```python
from build123d import *

# Parameters (mm, degrees)
F1_DEPTH = 5.842


with BuildPart() as f1:
    # F0 (on Top) → F1 (new body)
    with BuildSketch(Plane.XY):
        with BuildLine():
            Line((95.142507, 46.804437), (-38.207493, 46.804437))
            ThreePointArc((-38.207493, 46.804437), (-42.697621, 44.944565), (-44.557493, 40.454437))
            Line((-44.557493, 40.454437), (-44.557493, 27.754437))
            ThreePointArc((-44.557493, 27.754437), (-42.697621, 23.264309), (-38.207493, 21.404437))
            Line((-38.207493, 21.404437), (95.142507, 21.404437))
            Line((95.142507, 21.404437), (95.142507, 8.704437))
            Line((95.142507, 8.704437), (-38.207493, 8.704437))
            ThreePointArc((-38.207493, 8.704437), (-42.697621, 6.844565), (-44.557493, 2.354437))
            Line((-44.557493, 2.354437), (-44.557493, -10.345563))
            ThreePointArc((-44.557493, -10.345563), (-42.697621, -14.835691), (-38.207493, -16.695563))
            Line((-38.207493, -16.695563), (95.142507, -16.695563))
            Line((95.142507, -16.695563), (95.142507, -29.395563))
            Line((95.142507, -29.395563), (101.492507, -29.395563))
            Line((101.492507, -29.395563), (101.492507, 59.504437))
            Line((101.492507, 59.504437), (95.142507, 59.504437))
            Line((95.142507, 59.504437), (95.142507, 46.804437))
        make_face()
    extrude(amount=F1_DEPTH)


solid = f1.part
```
Geometry check sheet. Reference: the model listing, model coordinates, mm. A direction names the side the tool comes from. Round coordinates to 2 decimals unless told otherwise and drop trailing zeros. Loops run counter-clockwise (first coordinate to the right, second up) from the corner with the lowest first, then second, coordinate; pieces in that order, holes last. Notation, with made-up numbers: (-22.5, -12) - (5.5, -12) arc R27 ccw to (5.5, 14) - close; hole circle Ø4 at (75, 55.25). An arc over 180 degrees is marked (long way). Write each question's results on one line, items separated by ' | '. Start each with the question number.
Q1. Release check for a two-part mould opening along Y. For faces 1 (the cylindrical face through (-42.65, 6.89, 2.88)), 2 (the flat face through (27, 26, 0)), 3 (the flat face through (98, -29.396, 3)) record: +Y half, -Y half, draft (parallel to the pull), parting line (faces both ways), or undercut.
Q2. Cross-section at C-C on y = 51. Enter the section's corners in (x, z), and give its area (3 significant figures).
Q3. Cross-section at B-B on z = 3.9. Enter the section's corners in (x, y).
Q4. Gauge pin test, flat ends, axial feed: P1, Ø2, axis at x = 33, z = 5, coming from the -Y side; P2, Ø3, axis at y = 14, z = 3.5, coming from the -X side. Record the tip position at first contact, or that the pin passes through.
Q5. Thickness scan on line 1 (Y direction, x = 86.5, z = 4.85); line 2 (X direction, y = 11.5, z = 2.05); line 3 (X direction, y = 22, z = 1.3). Record the ranges inside material, lowest first. Write a range as [from, to].
Q6. Access from +Z, -Z, +X, -X, +Y, -Y to the whole of each face (thin tool, end or side, straight path). Record for faces 4 (the flat face through (-44.557, -4, 3)), 5 (the flat face through (29, 46.804, 3)), 6 (the cylindrical face through (-42.747, 23.314, 2.88)), 7 (the flat face through (95.143, -23, 3)).
Q7. Cross-section at A-A on x = 33.5. Enter the section's corners in (y, z), and give its area (3 significant figures).
Answers below:
1) face 1: undercut | face 2: draft | face 3: -Y half
2) outline: (95.14, 0) - (101.49, 0) - (101.49, 5.84) - (95.14, 5.84) - close | area: 37.1 mm²
3) outline: (-44.56, -10.35) arc R6.35 ccw to (-38.21, -16.7) - (95.14, -16.7) - (95.14, -29.4) - (101.49, -29.4) - (101.49, 59.5) - (95.14, 59.5) - (95.14, 46.8) - (-38.21, 46.8) arc R6.35 ccw to (-44.56, 40.45) - (-44.56, 27.75) arc R6.35 ccw to (-38.21, 21.4) - (95.14, 21.4) - (95.14, 8.7) - (-38.21, 8.7) arc R6.35 ccw to (-44.56, 2.35) - close
4) P1: stops at y = -16.7 | P2: stops at x = 95.14
5) line 1: y = [-16.7, 8.7], [21.4, 46.8] | line 2: x = [95.14, 101.49] | line 3: x = [-40.89, 101.49]
6) face 4: +Z, -Z, -X, +Y, -Y | face 5: +Z, -Z, -X, +Y | face 6: +Z, -Z, -X | face 7: +Z, -Z, -X, -Y
7) outline: (-16.7, 0) - (8.7, 0) - (8.7, 5.84) - (-16.7, 5.84) - close; (21.4, 0) - (46.8, 0) - (46.8, 5.84) - (21.4, 5.84) - close | area: 297 mm²
